from build123d import *

# Parameters (mm, degrees)
SKETCH1_R           = 29
SKETCH1_R_2         = 10
BOSS_EXTRUDE1_DEPTH = 2.54


with BuildPart() as part:
    # Sketch1 → Boss-Extrude1 (new body)
    with BuildSketch(Plane(origin=(0, 0, 0), x_dir=(1, 0, 0), z_dir=(0, 1, 0))):
        Circle(SKETCH1_R)
        Circle(SKETCH1_R_2, mode=Mode.SUBTRACT)
        with BuildLine():
            Line((70, 29), (0, 29))
            ThreePointArc((0, 29), (20.506096654, 20.506096654), (29, 0))
            ThreePointArc((29, 0), (20.506096654, -20.506096654), (0, -29))
            Line((0, -29), (70, -29))
            ThreePointArc((70, -29), (88.459414942, -22.366269246), (98.47367205, -5.5))
            Line((98.47367205, -5.5), (70, -5.5))
            ThreePointArc((70, -5.5), (64.5, 0), (70, 5.5))
            Line((70, 5.5), (98.47367205, 5.5))
            ThreePointArc((98.47367205, 5.5), (88.459414942, 22.366269246), (70, 29))
        make_face()
        with BuildLine():
            Line((88.940140067, -14.5), (48.940140067, -14.5))
            ThreePointArc((48.940140067, -14.5), (46.940140067, -12.5), (48.940140067, -10.5))
            Line((48.940140067, -10.5), (88.940140067, -10.5))
            ThreePointArc((88.940140067, -10.5), (90.354353629, -11.085786438), (90.940140067, -12.5))
            ThreePointArc((90.940140067, -12.5), (90.354353629, -13.914213562), (88.940140067, -14.5))
        make_face(mode=Mode.SUBTRACT)
        with BuildLine():
            Line((88.940140067, 10.5), (48.940140067, 10.5))
            ThreePointArc((48.940140067, 10.5), (46.940140067, 12.5), (48.940140067, 14.5))
            Line((48.940140067, 14.5), (88.940140067, 14.5))
            ThreePointArc((88.940140067, 14.5), (90.354353629, 13.914213562), (90.940140067, 12.5))
            ThreePointArc((90.940140067, 12.5), (90.354353629, 11.085786438), (88.940140067, 10.5))
        make_face(mode=Mode.SUBTRACT)
    extrude(amount=BOSS_EXTRUDE1_DEPTH)


solid = part.part
The model under review builds one solid part; all positions refer to its coordinate system, in mm. A direction names the side the tool comes from. Give positions to 0.01 mm unless a question says otherwise; leave off trailing zeros. Write each loop counter-clockwise with the first axis right and the second up, starting at its lowest first coordinate (ties: lowest second). Pieces come first, ordered by that corner, then holes.
1. Add section A-A, the plane x = 61.5. Write out the cut boundary in (y, z).
2. Draft analysis for pull direction Z (two halves, no side actions). For faces 4 (the flat face through (35, 1, -29)), 5 (the cylindrical face through (64.5, 1.3, 0.1)), 6 (the flat face through (34, 0, 0)), state which applies: +Z half, -Z half, draft (parallel to the pull), parting line (faces both ways), or undercut.
3. Add section C-C, the plane z = 3. Write out the cut boundary in (x, y), plus the area to 3 significant figures.
4. Wall thickness on L1, parallel to X at y = 0.7, z = 0; L2, parallel to X at y = 0.8, z = -4; L3, parallel to Z at x = 8.5, y = 1.8: over which ranges is each line inside the solid? List them lowest first.
5. Add section D-D, the plane z = 20. Write out the cut boundary in (x, y), plus the area to 3 significant figures.
6. Tool access review of faces 1 (the cylindrical face through (88.243, 1.252, 22.544)), 2 (the flat face through (84, 1, -5.5)), 3 (the flat face through (69, 1, -10.5)): name each direction out of +Z, -Z, +X, -X, +Y, -Y from which nothing blocks a thin tool from reaching the whole face with its end or side.
7. For P1, Ø1.3, axis at x = 76, y = 1, coming from the -Z side; P2, Ø0.8, axis at x = 89.5, y = 0.5, coming from the -Z side; P3, Ø1.3, axis at x = 74, y = 1, coming from the -Z side; P4, Ø16, axis at x = 0, z = 0, coming from the -Y side, all flat-tipped, find the tip position at first contact; note any pin that passes through.
8. Add section B-B, the plane y = 1.8. Write out the cut boundary in (x, z).
Worked answers:
1. outline: (0, -29) - (2.54, -29) - (2.54, -14.5) - (0, -14.5) - close; (0, -10.5) - (2.54, -10.5) - (2.54, 10.5) - (0, 10.5) - close; (0, 14.5) - (2.54, 14.5) - (2.54, 29) - (0, 29) - close
2. face 4: -Z half
2. face 5: undercut
2. face 6: draft
3. outline: (-28.84, 0) - (-9.54, 0) - (-9.54, 2.54) - (-28.84, 2.54) - close; (9.54, 0) - (65.39, 0) - (65.39, 2.54) - (9.54, 2.54) - close
3. area: 191 mm2
4. L1: x = -29 to -10, 10 to 64.5
4. L2: x = -28.72 to -9.17, 9.17 to 66.23
4. L3: z = -29 to -5.27, 5.27 to 29
5. outline: (-21, 0) - (91, 0) - (91, 2.54) - (-21, 2.54) - close
5. area: 284 mm2
6. face 1: +Z, +X, +Y, -Y
6. face 2: +X, +Y, -Y
6. face 3: +Y, -Y
7. P1: stops at z = -28.5
7. P2: stops at z = -21.82
7. P3: stops at z = -28.81
7. P4: passes through
8. outline: (0, -29) - (70, -29) arc R29 ccw to (98.47, -5.5) - (70, -5.5) arc R5.5 cw to (70, 5.5) - (98.47, 5.5) arc R29 ccw to (70, 29) - (0, 29) arc R29 ccw to start; hole circle Ø20 at (0, 0); hole (48.94, -14.5) - (88.94, -14.5) arc R2 ccw to (88.94, -10.5) - (48.94, -10.5) arc R2 ccw to start; hole (48.94, 10.5) - (88.94, 10.5) arc R2 ccw to (88.94, 14.5) - (48.94, 14.5) arc R2 ccw to start
